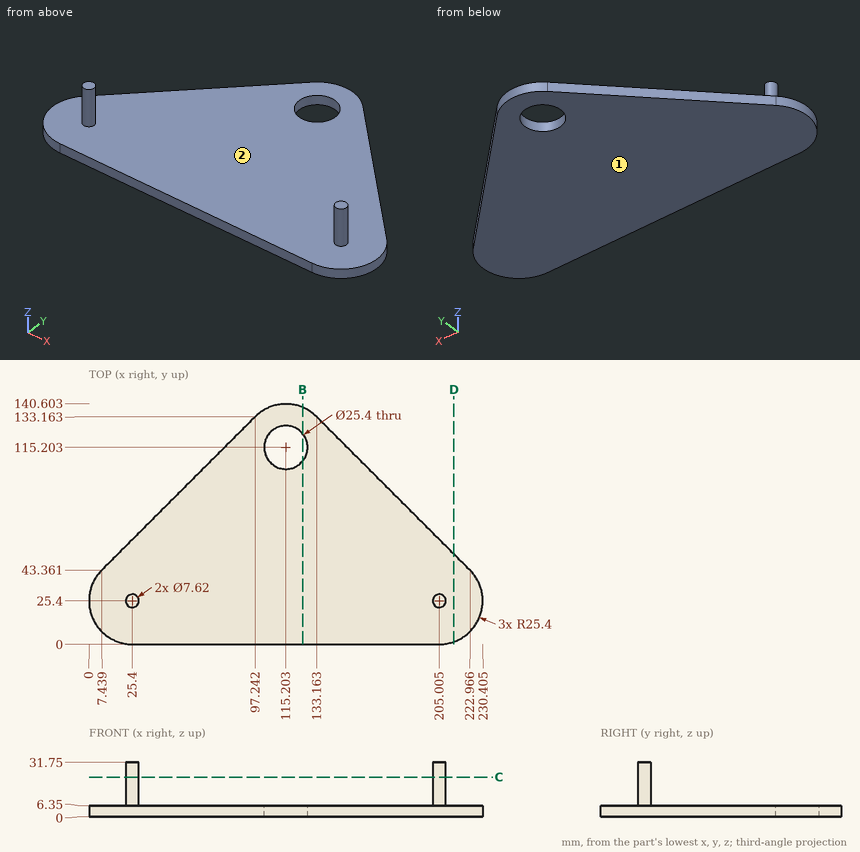
For this review, use the dimensioned drawing (mm, ordinates from the lowest corner) and the shaded views. Give positions to 0.01 mm unless a question says otherwise; leave off trailing zeros. Write each loop counter-clockwise with the first axis right and the second up, starting at its lowest first coordinate (ties: lowest second). Pieces come first, ordered by that corner, then holes. Notation, with made-up numbers: M 44.5,-16.75 L 52.5,-16.75 A26 ccw 52.5,17.25 Z; hole C 79.5,-27.75 d5. An arc over 180 degrees is marked long. Answer as a JSON object with one key per item and string values. Group by question number.
1) Mouldability with a two-part tool opening along Z and no side actions: class the marked faces 1 and 2 as released by +Z, released by -Z, zero draft, split by the parting line, or undercut.
2) We need section B-B (x = 125). Give the boundary of the cut face in (y, z).
3) We need section C-C (z = 23). Give the boundary of the cut face in (x, y) (1 decimal).
4) For line 1 along Z through (x, y) = (110.5, 89.5); line 2 along X through (y, z) = (94.5, 6) (1 decimal); line 3 along X through (y, z) = (38.5, 2.5) (1 decimal), list the stretches that pass through material, from the lowest coordinate up.
5) Clearance check with flat-ended pins moving along their axes: pin 1 Ø3 at (x, y) = (115.5, 27) entering from +Z; pin 2 Ø2 at (x, y) = (143.5, 38.5) entering from -Z. State where each tip first meets the part, or that it passes through.
6) We need section D-D (x = 213.5). Give the boundary of the cut face in (y, z).
Answer key:
{
 "1": {"face 1": "released by -Z", "face 2": "released by +Z"},
 "2": {"outline": "M 0,0 L 107.12,0 L 107.12,6.35 L 0,6.35 Z; M 123.28,0 L 138.64,0 L 138.64,6.35 L 123.28,6.35 Z"},
 "3": {"outline": "C 25.4,25.4 d7.6; C 205,25.4 d7.6"},
 "4": {"line 1": "z = 0 to 6.35", "line 2": "x = 58.6 to 171.8", "line 3": "x = 3.6 to 226.8"},
 "5": {"pin 1": "stops at z = 6.35", "pin 2": "stops at z = 0"},
 "6": {"outline": "M 1.46,0 L 52.83,0 L 52.83,6.35 L 1.46,6.35 Z"}
}
